from build123d import *

# Parameters (mm, degrees)
SKETCH_W     = 42.3
SKETCH_H     = 48.3
SKETCH_R     = 1.6
SKETCH_R_2   = 12
PAD_DEPTH    = 3
SKETCH001_W  = 42.3
SKETCH001_H  = 3
PAD001_DEPTH = 34
SKETCH002_R  = 1.5
POCKET_DEPTH = 48.301


with BuildPart() as part:
    # Sketch → Pad (new body)
    with BuildSketch(Plane.XY):
        with Locations((21.15, 24.15)):
            Rectangle(SKETCH_W, SKETCH_H)
        with Locations((5.65, 36.65)):
            Circle(SKETCH_R, mode=Mode.SUBTRACT)
        with Locations((36.65, 36.65)):
            Circle(SKETCH_R, mode=Mode.SUBTRACT)
        with Locations((5.65, 5.65)):
            Circle(SKETCH_R, mode=Mode.SUBTRACT)
        with Locations((36.65, 5.65)):
            Circle(SKETCH_R, mode=Mode.SUBTRACT)
        with Locations((21.15, 21.15)):
            Circle(SKETCH_R_2, mode=Mode.SUBTRACT)
    extrude(amount=PAD_DEPTH)

    # Sketch001 → Pad001 (new body)
    with BuildSketch(Plane(origin=(0, 0, 0), x_dir=(1, 0, 0), z_dir=(0, 0, -1))):
        with Locations((21.15, -46.8)):
            Rectangle(SKETCH001_W, SKETCH001_H)
    extrude(amount=PAD001_DEPTH)

    # Sketch002 → Pocket (cut, through all)
    with BuildSketch(Plane(origin=(0, 48.3, 0), x_dir=(-1, 0, 0), z_dir=(0, 1, 0))):
        with Locations((-30.2, -8)):
            Circle(SKETCH002_R)
        with Locations((-12.1, -8)):
            Circle(SKETCH002_R)
        with Locations((-30.2, -26)):
            Circle(SKETCH002_R)
        with Locations((-12.1, -26)):
            Circle(SKETCH002_R)
    extrude(amount=-POCKET_DEPTH, mode=Mode.SUBTRACT)


solid = part.part
The listing builds one solid part. Answer for the finished solid, in the listing's coordinates (mm). A direction names the side the tool comes from. Give positions to 0.01 mm unless a question says otherwise; leave off trailing zeros. Loops run counter-clockwise (first coordinate to the right, second up) from the corner with the lowest first, then second, coordinate; pieces in that order, holes last.
Item 1: A tool of negligible diameter and unlimited length cuts with its end or side. For faces 4 (the cylindrical face through (28.814, 46.821, -8.575)), 5 (the flat face through (16, 33, 0)), from which of +Z, -Z, +X, -X, +Y, -Y can it reach the whole face along a straight path? Write none if from no direction.
Derived:
face 4: +Y, -Y
face 5: -Z, +X, -X, -Y
Item 2: Each of these flat-tipped pins is pushed along its axis until it touches: pin 1 Ø3.5 at (x, y) = (36.65, 36.65) entering from -Z; pin 2 Ø5 at (x, z) = (12.1, -26) entering from -Y. Where does it stop, or does it pass through?
Derived:
pin 1: stops at z = 0
pin 2: stops at y = 45.3
Item 3: Determine the mould class of faces 1 (the cylindrical face through (35.38, 35.68, 1.48)), 2 (the flat face through (21, 45.3, -17)), 3 (the cylindrical face through (29.394, 46.821, -24.735)) for opening direction Y: +Y half, -Y half, draft (parallel to the pull), parting line (faces both ways), or undercut.
Derived:
face 1: undercut
face 2: -Y half
face 3: draft
Item 4: A cutting plane is placed at B-B (x = 21.15). Give the vertices of the cut face in (y, z).
Derived:
outline: (0, 0) - (9.15, 0) - (9.15, 3) - (0, 3) - close; (33.15, 0) - (45.3, 0) - (45.3, -34) - (48.3, -34) - (48.3, 3) - (33.15, 3) - close
Item 5: A cutting plane is placed at C-C (z = -26). Give the vertices of the cut face in (x, y), then the cut area to 3 significant figures.
Derived:
outline: (0, 45.3) - (10.6, 45.3) - (10.6, 48.3) - (0, 48.3) - close; (13.6, 45.3) - (28.7, 45.3) - (28.7, 48.3) - (13.6, 48.3) - close; (31.7, 45.3) - (42.3, 45.3) - (42.3, 48.3) - (31.7, 48.3) - close
area: 109 mm2
Item 6: Find the intervals of material crossed by line 1 along Z through (x, y) = (12, 47); line 2 along X through (y, z) = (21, 1); line 3 along Y through (x, z) = (16, -3), in increasing order.
Derived:
line 1: z = -34 to -27.5, -24.5 to -9.5, -6.5 to 3
line 2: x = 0 to 9.15, 33.15 to 42.3
line 3: y = 45.3 to 48.3
Item 7: A cutting plane is placed at D-D (x = 36.65). Give the vertices of the cut face in (y, z), then the cut area to 3 significant figures.
Derived:
outline: (0, 0) - (4.05, 0) - (4.05, 3) - (0, 3) - close; (7.25, 0) - (35.05, 0) - (35.05, 3) - (7.25, 3) - close; (38.25, 0) - (45.3, 0) - (45.3, -34) - (48.3, -34) - (48.3, 3) - (38.25, 3) - close
area: 228 mm2
Item 8: A cutting plane is placed at A-A (y = 21.15). Give the vertices of the cut face in (x, z).
Derived:
outline: (0, 0) - (9.15, 0) - (9.15, 3) - (0, 3) - close; (33.15, 0) - (42.3, 0) - (42.3, 3) - (33.15, 3) - close
